The model under review builds one solid part; all positions refer to its coordinate system, in mm. Give positions to 0.01 mm unless a question says otherwise; leave off trailing zeros. Order: outer loops, then holes, each group sorted by start corner. A loop starts at its lowest first (then second) coordinate and runs counter-clockwise, first axis right, second up.
```python
from build123d import *

# Parameters (mm, degrees)
F0_R     = 7.9375
F1_DEPTH = 12.7


with BuildPart() as f1:
    # F0 (on Top) → F1 (new body)
    with BuildSketch(Plane.XY):
        with BuildLine():
            ThreePointArc((0.977976, 15.844847), (0.407007, 15.117656), (0, 14.2875))
            ThreePointArc((0, 14.2875), (-0.407007, 15.117656), (-0.977976, 15.844847))
            Line((-0.977976, 15.844847), (-2.49475, 15.751229))
            Line((-2.49475, 15.751229), (-3.966216, 15.371557))
            ThreePointArc((-3.966216, 15.371557), (-4.284526, 14.503517), (-4.41508, 13.58822))
            ThreePointArc((-4.41508, 13.58822), (-5.058699, 14.251973), (-5.826438, 14.767134))
            Line((-5.826438, 14.767134), (-7.240045, 14.209389))
            Line((-7.240045, 14.209389), (-8.522168, 13.393591))
            ThreePointArc((-8.522168, 13.393591), (-8.55666, 12.469673), (-8.397982, 11.55883))
            ThreePointArc((-8.397982, 11.55883), (-9.215211, 11.991208), (-10.104567, 12.243911))
            Line((-10.104567, 12.243911), (-11.276635, 11.276635))
            Line((-11.276635, 11.276635), (-12.243911, 10.104567))
            ThreePointArc((-12.243911, 10.104567), (-11.991208, 9.215211), (-11.55883, 8.397982))
            ThreePointArc((-11.55883, 8.397982), (-12.469673, 8.55666), (-13.393591, 8.522168))
            Line((-13.393591, 8.522168), (-14.209389, 7.240045))
            Line((-14.209389, 7.240045), (-14.767134, 5.826438))
            ThreePointArc((-14.767134, 5.826438), (-14.251973, 5.058699), (-13.58822, 4.41508))
            ThreePointArc((-13.58822, 4.41508), (-14.503517, 4.284526), (-15.371557, 3.966216))
            Line((-15.371557, 3.966216), (-15.751229, 2.49475))
            Line((-15.751229, 2.49475), (-15.844847, 0.977976))
            ThreePointArc((-15.844847, 0.977976), (-15.117656, 0.407007), (-14.2875, 0))
            ThreePointArc((-14.2875, 0), (-15.117656, -0.407007), (-15.844847, -0.977976))
            Line((-15.844847, -0.977976), (-15.751229, -2.49475))
            Line((-15.751229, -2.49475), (-15.371557, -3.966216))
            ThreePointArc((-15.371557, -3.966216), (-14.503517, -4.284526), (-13.58822, -4.41508))
            ThreePointArc((-13.58822, -4.41508), (-14.251973, -5.058699), (-14.767134, -5.826438))
            Line((-14.767134, -5.826438), (-14.209389, -7.240045))
            Line((-14.209389, -7.240045), (-13.393591, -8.522168))
            ThreePointArc((-13.393591, -8.522168), (-12.469673, -8.55666), (-11.55883, -8.397982))
            ThreePointArc((-11.55883, -8.397982), (-11.991208, -9.215211), (-12.243911, -10.104567))
            Line((-12.243911, -10.104567), (-11.276635, -11.276635))
            Line((-11.276635, -11.276635), (-10.104567, -12.243911))
            ThreePointArc((-10.104567, -12.243911), (-9.215211, -11.991208), (-8.397982, -11.55883))
            ThreePointArc((-8.397982, -11.55883), (-8.55666, -12.469673), (-8.522168, -13.393591))
            Line((-8.522168, -13.393591), (-7.240045, -14.209389))
            Line((-7.240045, -14.209389), (-5.826438, -14.767134))
            ThreePointArc((-5.826438, -14.767134), (-5.058699, -14.251973), (-4.41508, -13.58822))
            ThreePointArc((-4.41508, -13.58822), (-4.284526, -14.503517), (-3.966216, -15.371557))
            Line((-3.966216, -15.371557), (-2.49475, -15.751229))
            Line((-2.49475, -15.751229), (-0.977976, -15.844847))
            ThreePointArc((-0.977976, -15.844847), (-0.407007, -15.117656), (0, -14.2875))
            ThreePointArc((0, -14.2875), (0.407007, -15.117656), (0.977976, -15.844847))
            Line((0.977976, -15.844847), (2.49475, -15.751229))
            Line((2.49475, -15.751229), (3.966216, -15.371557))
            ThreePointArc((3.966216, -15.371557), (4.284526, -14.503517), (4.41508, -13.58822))
            ThreePointArc((4.41508, -13.58822), (5.058699, -14.251973), (5.826438, -14.767134))
            Line((5.826438, -14.767134), (7.240045, -14.209389))
            Line((7.240045, -14.209389), (8.522168, -13.393591))
            ThreePointArc((8.522168, -13.393591), (8.55666, -12.469673), (8.397982, -11.55883))
            ThreePointArc((8.397982, -11.55883), (9.215211, -11.991208), (10.104567, -12.243911))
            Line((10.104567, -12.243911), (11.276635, -11.276635))
            Line((11.276635, -11.276635), (12.243911, -10.104567))
            ThreePointArc((12.243911, -10.104567), (11.991208, -9.215211), (11.55883, -8.397982))
            ThreePointArc((11.55883, -8.397982), (12.469673, -8.55666), (13.393591, -8.522168))
            Line((13.393591, -8.522168), (14.209389, -7.240045))
            Line((14.209389, -7.240045), (14.767134, -5.826438))
            ThreePointArc((14.767134, -5.826438), (14.251973, -5.058699), (13.58822, -4.41508))
            ThreePointArc((13.58822, -4.41508), (14.503517, -4.284526), (15.371557, -3.966216))
            Line((15.371557, -3.966216), (15.751229, -2.49475))
            Line((15.751229, -2.49475), (15.844847, -0.977976))
            ThreePointArc((15.844847, -0.977976), (15.117656, -0.407007), (14.2875, 0))
            ThreePointArc((14.2875, 0), (15.117656, 0.407007), (15.844847, 0.977976))
            Line((15.844847, 0.977976), (15.751229, 2.49475))
            Line((15.751229, 2.49475), (15.371557, 3.966216))
            ThreePointArc((15.371557, 3.966216), (14.503517, 4.284526), (13.58822, 4.41508))
            ThreePointArc((13.58822, 4.41508), (14.251973, 5.058699), (14.767134, 5.826438))
            Line((14.767134, 5.826438), (14.209389, 7.240045))
            Line((14.209389, 7.240045), (13.393591, 8.522168))
            ThreePointArc((13.393591, 8.522168), (12.469673, 8.55666), (11.55883, 8.397982))
            ThreePointArc((11.55883, 8.397982), (11.991208, 9.215211), (12.243911, 10.104567))
            Line((12.243911, 10.104567), (11.276635, 11.276635))
            Line((11.276635, 11.276635), (10.104567, 12.243911))
            ThreePointArc((10.104567, 12.243911), (9.215211, 11.991208), (8.397982, 11.55883))
            ThreePointArc((8.397982, 11.55883), (8.55666, 12.469673), (8.522168, 13.393591))
            Line((8.522168, 13.393591), (7.240045, 14.209389))
            Line((7.240045, 14.209389), (5.826438, 14.767134))
            ThreePointArc((5.826438, 14.767134), (5.058699, 14.251973), (4.41508, 13.58822))
            ThreePointArc((4.41508, 13.58822), (4.284526, 14.503517), (3.966216, 15.371557))
            Line((3.966216, 15.371557), (2.49475, 15.751229))
            Line((2.49475, 15.751229), (0.977976, 15.844847))
        make_face()
        Circle(F0_R, mode=Mode.SUBTRACT)
    extrude(amount=F1_DEPTH)


solid = f1.part
```
Item 1: Clearance check with flat-ended pins moving along their axes: pin 1 Ø1 at (y, z) = (5.5, 2.5) entering from -X; pin 2 Ø2 at (x, z) = (12.5, 8.5) entering from +Y; pin 3 Ø1 at (x, z) = (11, 8.5) entering from -Y. State where each tip first meets the part, or that it passes through.
Values found:
pin 1: stops at x = -14.77
pin 2: stops at y = 11.01
pin 3: stops at y = -11.92
Item 2: Take a section at C-C (y = 13). Give the boundary of the cut face in (x, z), and give its area (3 significant figures).
Values found:
outline: (-8.56, 0) - (8.56, 0) - (8.56, 12.7) - (-8.56, 12.7) - close
area: 217 mm2
Item 3: Draft analysis for pull direction X (two halves, no side actions). For faces 1 (the flat face through (-13.796, 7.89, 6.261)), 2 (the flat face through (-7.3, 3.7, 12.7)), 3 (the cylindrical face through (0.4, -15.11, 6.26)), state which applies: released by +X, released by -X, zero draft, split by the parting line, or undercut.
Values found:
face 1: released by -X
face 2: zero draft
face 3: undercut
Item 4: Take a section at D-D (x = -10.5). Give the boundary of the cut face in (y, z), and give its area (3 significant figures).
Values found:
outline: (-11.92, 0) - (11.92, 0) - (11.92, 12.7) - (-11.92, 12.7) - close
area: 303 mm2
Item 5: For line 1 (Y direction, x = -14, z = 7.75); line 2 (Y direction, x = -0.5, z = 8); line 3 (Y direction, x = -2, z = 2), list the stretches that pass through material, from the lowest coordinate up.
Values found:
line 1: y = -7.57 to -4.78, -4.38 to 4.38, 4.78 to 7.57
line 2: y = -15.26 to -7.92, 7.92 to 15.26
line 3: y = -15.78 to -7.68, 7.68 to 15.78
Item 6: Take a section at B-B (y = 6.5). Give the boundary of the cut face in (x, z), and give its area (3 significant figures).
Values found:
outline: (-14.5, 0) - (-4.56, 0) - (-4.56, 12.7) - (-14.5, 12.7) - close; (4.56, 0) - (14.5, 0) - (14.5, 12.7) - (4.56, 12.7) - close
area: 253 mm2
Item 7: Take a section at A-A (x = 0.5). Give the boundary of the cut face in (y, z), and give its area (3 significant figures).
Values found:
outline: (-15.26, 0) - (-7.92, 0) - (-7.92, 12.7) - (-15.26, 12.7) - close; (7.92, 0) - (15.26, 0) - (15.26, 12.7) - (7.92, 12.7) - close
area: 186 mm2
